Part model, mm, in its own coordinate system. Face numbers are marked on the shaded views. A direction names the side the tool comes from. Give positions to 0.01 mm unless a question says otherwise; leave off trailing zeros. Order: outer loops, then holes, each group sorted by start corner. A loop starts at its lowest first (then second) coordinate and runs counter-clockwise, first axis right, second up. Notation, with made-up numbers: M 81,65.25 L 115,65.25 A29 cw 115,90.25 Z; hole C -24.5,-17 d5. An arc over 180 degrees is marked long. Return JSON: item names as keys, results as strings.
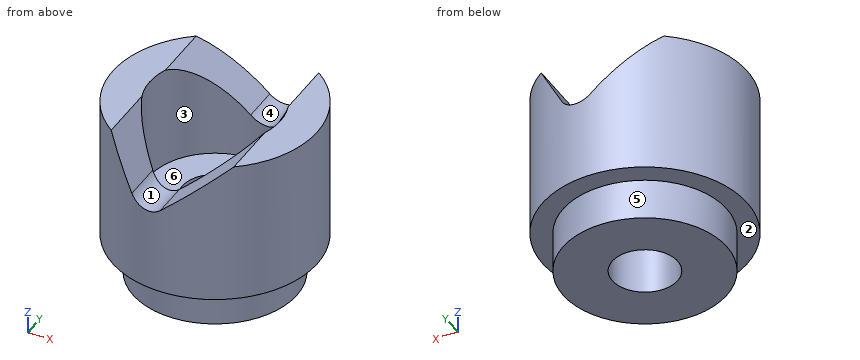
from build123d import *

# Parameters (mm, degrees)
PAD002_DEPTH    = 10
PAD001_DEPTH    = 12
SKETCH_R        = 5
SKETCH_R_2      = 1.6
PAD_DEPTH       = 9
SKETCH001_R     = 3.2
POCKET_DEPTH    = 5
SKETCH002_R     = 5
SKETCH002_R_2   = 4
POCKET001_DEPTH = 2
FILLET_R        = 1


with BuildPart() as pad002:
    # Sketch004 → Pad002 (new body)
    with BuildSketch(Plane.XZ):
        Polygon((-3, 9), (1, 5.5), (3, 9), align=None)
    extrude(amount=-PAD002_DEPTH)


with BuildPart() as pad001:
    # Sketch003 → Pad001 (new body)
    with BuildSketch(Plane.XZ):
        Polygon((-3, 9), (-1, 5.5), (3, 9), align=None)
    extrude(amount=PAD001_DEPTH)


with BuildPart() as fillet_body:
    # Sketch → Pad (new body)
    with BuildSketch(Plane.XY):
        Circle(SKETCH_R)
        Circle(SKETCH_R_2, mode=Mode.SUBTRACT)
    extrude(amount=PAD_DEPTH)

    # Sketch001 → Pocket (cut)
    with BuildSketch(Plane.XY.offset(9)):
        Circle(SKETCH001_R)
    extrude(amount=-POCKET_DEPTH, mode=Mode.SUBTRACT)

    # Sketch002 → Pocket001 (cut)
    with BuildSketch(Plane(origin=(0, 0, 0), x_dir=(1, 0, 0), z_dir=(0, 0, -1))):
        Circle(SKETCH002_R)
        Circle(SKETCH002_R_2, mode=Mode.SUBTRACT)
    extrude(amount=-POCKET001_DEPTH, mode=Mode.SUBTRACT)

    # Cut: cut Pad001
    add(pad001.part, mode=Mode.SUBTRACT)

    # Cut001: cut Pad002
    add(pad002.part, mode=Mode.SUBTRACT)

    # Fillet
    fillet_edges = [fillet_body.edges().sort_by_distance(p)[0] for p in [
        (1, 3.969358, 5.5),
        (-1, -3.969358, 5.5),
    ]]
    fillet(fillet_edges, radius=FILLET_R)


solid = fillet_body.part
Q1. Pin check, flat tips, straight feed: pin 1 (3.5 mm diameter, centred on x = 0, y = 0, fed in from +Z); pin 2 (1.5 mm diameter, centred on x = -2, z = 3.5, fed in from -Y); pin 3 (1.5 mm diameter, centred on y = -2.5, z = 7.5, fed in from +X). Stop position of each tip, or through.
Established:
{"pin 1": "stops at z = 4", "pin 2": "stops at y = -4.84", "pin 3": "stops at x = 4.68"}
Q2. Band-saw the part on A-A (y = 0). Give the cut face in (x, z).
Established:
{"outline": "M -5,2 L -4,2 L -4,0 L -1.6,0 L -1.6,4 L -3.2,4 L -3.2,9 L -5,9 Z; M 1.6,0 L 4,0 L 4,2 L 5,2 L 5,9 L 3.2,9 L 3.2,4 L 1.6,4 Z"}
Q3. 3-axis set-ups, long thin cutter, end or side, ignore diameter. For the marked faces 1, 2 and 3: which of +Z, -Z, +X, -X, +Y, -Y reach the whole face in a straight line?
Established:
{"face 1": "+Z, -Y", "face 2": "-Z", "face 3": "+Z"}
Q4. Two-plate mould, pull along Y, no slides. Class the marked faces 4, 5 and 6: +Y half, -Y half, draft (parallel to the pull), parting line (faces both ways), or undercut.
Established:
{"face 4": "draft", "face 5": "parting line", "face 6": "undercut"}
Q5. Band-saw the part on C-C (z = 7.75). Give the cut face in (x, y), then the cut area to 3 significant figures.
Established:
{"outline": "M -2.29,-4.45 L -2.29,-2.24 A3.2 cw -1.57,2.79 L -1.57,4.75 A5 ccw Z; M 1.57,-4.75 A5 ccw 2.29,4.45 L 2.29,2.24 A3.2 cw 1.57,-2.79 Z", "area": "31.8 mm²"}
Q6. Band-saw the part on B-B (x = -0.25). Give the cut face in (y, z).
Established:
{"outline": "M -4.99,2 L -3.99,2 L -3.99,0 L -1.58,0 L -1.58,4 L -3.19,4 L -3.19,6.19 L -4.99,6.19 Z; M 1.58,0 L 3.99,0 L 3.99,2 L 4.99,2 L 4.99,6.59 L 3.19,6.59 L 3.19,4 L 1.58,4 Z"}
Q7. Probe line 1 along Y through (x, z) = (0, 1.9); line 2 along Y through (x, z) = (0, 2.5); line 3 along X through (y, z) = (0, 7.6). List the from-to ranges inside material, lowest first.
Established:
{"line 1": "y = -4 to -1.6, 1.6 to 4", "line 2": "y = -5 to -1.6, 1.6 to 5", "line 3": "x = -5 to -3.2, 3.2 to 5"}
Q8. Band-saw the part on D-D (z = 4.25). Give the cut face in (x, y).
Established:
{"outline": "C 0,0 d10; hole C 0,0 d6.4"}
